from build123d import *

# Parameters (mm, degrees)
BOSS_EXTRUDE1_DEPTH = 10
SKETCH2_R           = 1
SKETCH2_W           = 116.84899
SKETCH2_H           = 75.7696
BOSS_EXTRUDE2_DEPTH = 1
CAVITY1_START       = 1.833256049
CAVITY1_OUTLINE_W   = 1
CAVITY1_OUTLINE_H   = 71.506597146
CAVITY1_DEPTH       = 8.166743951
FILLET1_R           = 3
FILLET2_R           = 3
FILLET3_R           = 3


# Read off the part's stored shape, not the designer's step: Cavity1
with BuildPart() as part:
    # Sketch1 → Boss-Extrude1 (new body)
    with BuildSketch(Plane.XY):
        with BuildLine():
            Line((-67.723179308, 39.023349276), (57.135904391, 39.023349276))
            ThreePointArc((57.135904391, 39.023349276), (60.664300974, 37.561839558), (62.125810692, 34.033442975))
            Line((62.125810692, 34.033442975), (62.125810692, -49.746250724))
            ThreePointArc((62.125810692, -49.746250724), (60.661344598, -53.28178463), (57.125810692, -54.746250724))
            Line((57.125810692, -54.746250724), (-67.723179308, -54.746250724))
            ThreePointArc((-67.723179308, -54.746250724), (-71.258713213, -53.28178463), (-72.723179308, -49.746250724))
            Line((-72.723179308, -49.746250724), (-72.723179308, 34.023349276))
            ThreePointArc((-72.723179308, 34.023349276), (-71.258713213, 37.558883182), (-67.723179308, 39.023349276))
        make_face()
        with BuildLine():
            Line((-67.723179308, 38.023349276), (57.135904391, 38.023349276))
            ThreePointArc((57.135904391, 38.023349276), (59.957194193, 36.854732777), (61.125810692, 34.033442975))
            Line((61.125810692, 34.033442975), (61.125810692, -49.746250724))
            ThreePointArc((61.125810692, -49.746250724), (59.954237817, -52.574677849), (57.125810692, -53.746250724))
            Line((57.125810692, -53.746250724), (-67.723179308, -53.746250724))
            ThreePointArc((-67.723179308, -53.746250724), (-70.551606432, -52.574677849), (-71.723179308, -49.746250724))
            Line((-71.723179308, -49.746250724), (-71.723179308, 34.023349276))
            ThreePointArc((-71.723179308, 34.023349276), (-70.551606432, 36.851776401), (-67.723179308, 38.023349276))
        make_face(mode=Mode.SUBTRACT)
    extrude(amount=BOSS_EXTRUDE1_DEPTH)

    # Sketch2 → Boss-Extrude2 (add)
    with BuildSketch(Plane.XY):
        with BuildLine():
            Line((-67.723179308, 38.023349276), (57.135904391, 38.023349276))
            ThreePointArc((57.135904391, 38.023349276), (59.957194193, 36.854732777), (61.125810692, 34.033442975))
            Line((61.125810692, 34.033442975), (61.125810692, -49.746250724))
            ThreePointArc((61.125810692, -49.746250724), (59.954237817, -52.574677849), (57.125810692, -53.746250724))
            Line((57.125810692, -53.746250724), (-67.723179308, -53.746250724))
            ThreePointArc((-67.723179308, -53.746250724), (-70.551606432, -52.574677849), (-71.723179308, -49.746250724))
            Line((-71.723179308, -49.746250724), (-71.723179308, 34.023349276))
            ThreePointArc((-71.723179308, 34.023349276), (-70.551606432, 36.851776401), (-67.723179308, 38.023349276))
        make_face()
        with Locations((-67.798179308, 34.314149276)):
            Circle(SKETCH2_R, mode=Mode.SUBTRACT)
        with Locations((-68.073179308, -49.962350724)):
            Circle(SKETCH2_R, mode=Mode.SUBTRACT)
        with Locations((57.254910692, -50.238050724)):
            Circle(SKETCH2_R, mode=Mode.SUBTRACT)
        with Locations((57.530010692, 34.311649276)):
            Circle(SKETCH2_R, mode=Mode.SUBTRACT)
        with Locations((-5.298684308, -7.861450724)):
            Rectangle(SKETCH2_W, SKETCH2_H, mode=Mode.SUBTRACT)
    extrude(amount=BOSS_EXTRUDE2_DEPTH)

    # Cavity1 outline → Cavity1 (cut)
    with BuildSketch(Plane.XY.offset(CAVITY1_START)):
        with Locations((61.625810692, -7.448622115)):
            Rectangle(CAVITY1_OUTLINE_W, CAVITY1_OUTLINE_H)
        with Locations((-72.223179308, -7.448622115)):
            Rectangle(CAVITY1_OUTLINE_W, CAVITY1_OUTLINE_H)
    extrude(amount=CAVITY1_DEPTH, mode=Mode.SUBTRACT)

    # Fillet1
    fillet1_edges = [part.edges().sort_by_distance(p)[0] for p in [
        (61.625810692, -43.201920688, 10),
        (-72.223179308, -43.201920688, 10),
        (-72.223179308, 28.304676458, 10),
        (61.625810692, 28.304676458, 10),
    ]]
    fillet(fillet1_edges, radius=FILLET1_R)

    # Fillet2
    fillet2_edges = [part.edges().sort_by_distance(p)[0] for p in [
        (-72.223179308, -43.201920688, 1.833256049),
        (-72.223179308, 28.304676458, 1.833256049),
        (61.625810692, -43.201920688, 1.833256049),
        (61.625810692, 28.304676458, 1.833256049),
    ]]
    fillet(fillet2_edges, radius=FILLET2_R)

    # Fillet3
    fillet3_edges = [part.edges().sort_by_distance(p)[0] for p in [
        (-63.723179308, -45.746250724, 0.5),
        (53.125810692, -45.746250724, 0.5),
        (53.125810692, 30.023349276, 0.5),
        (-63.723179308, 30.023349276, 0.5),
    ]]
    fillet(fillet3_edges, radius=FILLET3_R)


solid = part.part
Geometry: final body of the model. Coordinates: model frame, mm. A direction names the side the tool comes from. Round coordinates to 2 decimals unless told otherwise and drop trailing zeros. Loops run counter-clockwise (first coordinate to the right, second up) from the corner with the lowest first, then second, coordinate; pieces in that order, holes last. Notation, with made-up numbers: (48, 74) -> (60, 74) arc R25 cw to (60, 99) -> close; hole circle Ø5 at (-36.75, -26). An arc over 180 degrees is marked (long way). One line per question, with ' | ' between items. Start each with the question number.
1. Section A-A on y = -22. Output: boundary loops of the cut face in (x, z), and give its area (3 significant figures).
2. Contact query for flat-ended pins moving along their axis: pin 1 (0.5 mm diameter, centred on x = 61.5, z = 6, fed in from -Y); pin 2 (1.1 mm diameter, centred on x = -72, z = 6, fed in from +Y); pin 3 (3 mm diameter, centred on x = -67.8, y = 34.31, fed in from +Z); pin 4 (1.5 mm diameter, centred on x = 13.5, y = 29.5, fed in from -Z). Output: stop coordinate, or through.
3. Section B-B on x = 18. Output: boundary loops of the cut face in (y, z).
4. Line query: line 1 along Y through (x, z) = (-41.5, 9); line 2 along X through (y, z) = (-42, 1.5); line 3 along Z through (x, y) = (-27, 33). Output: solid intervals per line, ascending. Write a range as [from, to].
5. Mould query, pull axis X, two halves, no side actions, for faces 1 (the face through (-72.723, -8.4, 1.6)), 2 (the face through (59.926, 36.886, 5.437)), 3 (the face through (61.63, -42.35, 2.74)). Classes: pulls with the +X half, pulls with the -X half, needs draft (parallel to the pull), parting line crosses it, or undercut.
6. Set-up query: faces 4 (the face through (61.63, -44.1, 9.14)), 5 (the face through (-5, 38.3, 10)), 6 (the face through (-71.723, -8.1, 1.5)), 7 (the face through (-4, 34, 0)), 8 (the face through (52.224, -44.891, 0.507)). Return all of +Z, -Z, +X, -X, +Y, -Y with unobstructed straight access to the full face (end or side cutting, diameter ignored); none if empty.
7. Section C-C on z = 3.5. Output: boundary loops of the cut face in (x, y), and give its area (3 significant figures).
Returned:
1) outline: (-72.72, 0) -> (-63.72, 0) -> (-63.72, 1) -> (-71.72, 1) -> (-71.72, 1.83) -> (-72.72, 1.83) -> close; (53.13, 0) -> (62.13, 0) -> (62.13, 1.83) -> (61.13, 1.83) -> (61.13, 1) -> (53.13, 1) -> close | area: 19.7 mm2
2) pin 1: stops at y = -52.57 | pin 2: stops at y = 37.36 | pin 3: stops at z = 1 | pin 4: stops at z = 0
3) outline: (-54.75, 0) -> (-45.75, 0) -> (-45.75, 1) -> (-53.75, 1) -> (-53.75, 10) -> (-54.75, 10) -> close; (30.02, 0) -> (39.02, 0) -> (39.02, 10) -> (38.02, 10) -> (38.02, 1) -> (30.02, 1) -> close
4) line 1: y = [-54.75, -53.75], [38.02, 39.02] | line 2: x = [-72.72, -71.72], [61.13, 62.13] | line 3: z = [0, 1]
5) face 1: pulls with the -X half | face 2: undercut | face 3: needs draft
6) face 4: +Z, +X, -X | face 5: +Z, +X, -X, +Y, -Y | face 6: +Z | face 7: -Z, +X, -X, +Y, -Y | face 8: +Z, -Z
7) outline: (-72.72, -49.75) arc R5 ccw to (-67.72, -54.75) -> (57.13, -54.75) arc R5 ccw to (62.13, -49.75) -> (62.13, -42.89) -> (61.13, -42.89) -> (61.13, -49.75) arc R4 cw to (57.13, -53.75) -> (-67.72, -53.75) arc R4 cw to (-71.72, -49.75) -> (-71.72, -42.89) -> (-72.72, -42.89) -> close; (-72.72, 27.99) -> (-71.72, 27.99) -> (-71.72, 34.02) arc R4 cw to (-67.72, 38.02) -> (57.14, 38.02) arc R3.99 cw to (61.13, 34.03) -> (61.13, 27.99) -> (62.13, 27.99) -> (62.13, 34.03) arc R4.99 ccw to (57.14, 39.02) -> (-67.72, 39.02) arc R5 ccw to (-72.72, 34.02) -> close | area: 304 mm2
